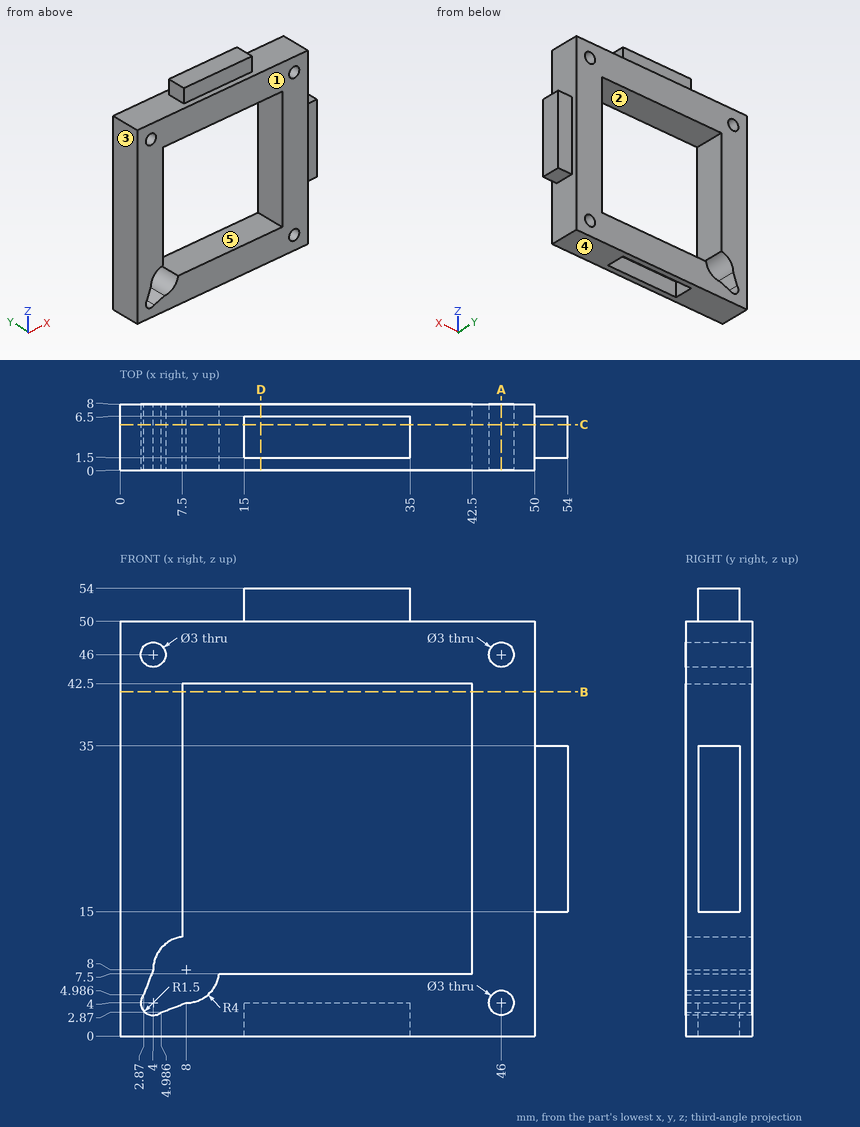
Can you work these out from the drawing? Everything is in mm from the part's minimum corner. A direction names the side the tool comes from. Coordinates: 2 decimals unless noted, no trailing zeros. Loops run counter-clockwise (first coordinate to the right, second up) from the corner with the lowest first, then second, coordinate; pieces in that order, holes last. Notation, with made-up numbers: M 13,12.25 L 23,12.25 A21 ccw 23,45.25 Z; hole C 75.5,41 d9. An arc over 180 degrees is marked long. One line per item, written item: value.
1. Imagine slicing it at C-C (y = 5.5). List the corners of the cut face in (x, z) for me.
Geometry says:
outline: M 0,0 L 15,0 L 15,4 L 35,4 L 35,0 L 50,0 L 50,15 L 54,15 L 54,35 L 50,35 L 50,50 L 35,50 L 35,54 L 15,54 L 15,50 L 0,50 Z; hole C 4,46 d3; hole M 2.87,4.99 A1.5 ccw 4.99,2.87 L 8,4 A4 ccw 11.97,7.5 L 42.5,7.5 L 42.5,42.5 L 7.5,42.5 L 7.5,11.97 A4 ccw 4,8 Z; hole C 46,4 d3; hole C 46,46 d3
2. Imagine slicing it at A-A (x = 46). List the corners of the cut face in (y, z) for me.
Geometry says:
outline: M 0,0 L 8,0 L 8,2.5 L 0,2.5 Z; M 0,5.5 L 8,5.5 L 8,44.5 L 0,44.5 Z; M 0,47.5 L 8,47.5 L 8,50 L 0,50 Z
3. Imagine slicing it at B-B (z = 41.5). List the corners of the cut face in (x, y) for me.
Geometry says:
outline: M 0,0 L 7.5,0 L 7.5,8 L 0,8 Z; M 42.5,0 L 50,0 L 50,8 L 42.5,8 Z
4. Will these pins go through, and if not, where does the flat tip stop? pin 1 Ø3 at (y, z) = (3, 3) entering from -X; pin 2 Ø2 at (y, z) = (5, 1.5) entering from +X; pin 3 Ø1.2 at (x, y) = (52, 3) entering from -Z; pin 4 Ø4.5 at (x, z) = (53, 28) entering from +Y.
Geometry says:
pin 1: stops at x = 0
pin 2: stops at x = 50
pin 3: stops at z = 15
pin 4: stops at y = 6.5
5. Please list where these lines run through material, in increasing order: probe 1 along X at (y, z) = (6.25, 14); probe 2 along X at (y, z) = (6, 46); probe 3 along X at (y, z) = (6, 32.5).
Geometry says:
probe 1: x = 0 to 7.5, 42.5 to 50
probe 2: x = 0 to 2.5, 5.5 to 44.5, 47.5 to 50
probe 3: x = 0 to 7.5, 42.5 to 54
6. Thinking about a two-plate mould opening in X: for the marked faces 1, 2 and 3, which applies, +X half, -X half, draft (parallel to the pull), parting line (faces both ways), or undercut?
Geometry says:
face 1: draft
face 2: undercut
face 3: -X half
7. Imagine slicing it at D-D (x = 17). List the corners of the cut face in (y, z) for me.
Geometry says:
outline: M 0,0 L 1.5,0 L 1.5,4 L 6.5,4 L 6.5,0 L 8,0 L 8,7.5 L 0,7.5 Z; M 0,42.5 L 8,42.5 L 8,50 L 6.5,50 L 6.5,54 L 1.5,54 L 1.5,50 L 0,50 Z
8. On a 3-axis mill with a long thin cutter (end or side, diameter ignored), from which of +Z, -Z, +X, -X, +Y, -Y can I reach the whole of each face in a straight line? I mean the marked faces 4 and 5. Say none if no direction works.
Geometry says:
face 4: -Z, +X, -X, +Y, -Y
face 5: +Y, -Y
